```python
from build123d import *

# Parameters (mm, degrees)
F1_DEPTH = 2.413
F2_R     = 10.922
F3_DEPTH = 1.524
F4_R     = 6.223
F4_R_2   = 1.27
F5_DEPTH = 12.065
F6_R     = 5.461
F6_R_2   = 1.524
F7_DEPTH = 1.27


with BuildPart() as f1:
    # F0 (on Top) → F1 (new body)
    with BuildSketch(Plane.XY):
        with BuildLine():
            Line((-16.002, -18.188851), (16.002, -18.188851))
            Line((16.002, -18.188851), (16.002, 18.188851))
            Line((16.002, 18.188851), (9.906, 18.188851))
            Line((9.906, 18.188851), (9.906, 4.600136))
            ThreePointArc((9.906, 4.600136), (5.875687, 9.206866), (0, 10.922))
            ThreePointArc((0, 10.922), (-5.875687, 9.206866), (-9.906, 4.600136))
            Line((-9.906, 4.600136), (-9.906, 18.188851))
            Line((-9.906, 18.188851), (-16.002, 18.188851))
            Line((-16.002, 18.188851), (-16.002, -18.188851))
        make_face()
    extrude(amount=F1_DEPTH)

    # F2 (on face) → F3 (join)
    with BuildSketch(Plane(origin=(0, 0, 0), x_dir=(1, 0, 0), z_dir=(0, 0, -1))):
        Circle(F2_R)
    extrude(amount=F3_DEPTH)

    # F4 (on face) → F5 (join)
    with BuildSketch(Plane(origin=(0, 0, -1.524), x_dir=(1, 0, 0), z_dir=(0, 0, -1))):
        Circle(F4_R)
        Circle(F4_R_2, mode=Mode.SUBTRACT)
    extrude(amount=F5_DEPTH)

    # F6 (on face) → F7 (join)
    with BuildSketch(Plane(origin=(0, 0, -13.589), x_dir=(1, 0, 0), z_dir=(0, 0, -1))):
        Circle(F6_R)
        Circle(F6_R_2, mode=Mode.SUBTRACT)
    extrude(amount=F7_DEPTH)


solid = f1.part
```
Part model, mm, in its own coordinate system. A direction names the side the tool comes from. Round coordinates to 2 decimals unless told otherwise and drop trailing zeros. Loops run counter-clockwise (first coordinate to the right, second up) from the corner with the lowest first, then second, coordinate; pieces in that order, holes last.
Item 1: 3-axis set-ups, long thin cutter, end or side, ignore diameter. For faces 1 (the face through (9.906, 11, 1)), 2 (the face through (-0.17, -1.26, -7.47)): which of +Z, -Z, +X, -X, +Y, -Y reach the whole face in a straight line?
Item 2: Cut at A-A, the plane y = 0. Give the cut face in (x, z), then the cut area to 3 significant figures.
Item 3: Mould opens along X. For faces 3 (the face through (5, 5, -1.524)), 4 (the face through (-0.2, -1.51, -14.22)), 5 (the face through (-1.349, 6.075, -7.472)) say: +X half, -X half, draft (parallel to the pull), parting line (faces both ways), or undercut.
Item 4: Cut at C-C, the plane x = 4.5. Give the cut face in (y, z).
Item 5: Drop flat-ended pins along their axis: P1, Ø0.9, axis at x = 0, y = 0.5, coming from the -Z side; P2, Ø3, axis at x = 7, z = -6.5, coming from the +Y side; P3, Ø3, axis at y = -6, z = -5.5, coming from the -X side. Give the stop position or say it passes through.
Item 6: Cut at B-B, the plane y = 15. Give the cut face in (x, z).
Item 7: Cut at D-D, the plane y = 8.5. Give the cut face in (x, z).
Item 8: Drill centre lines: line 1 (X direction, y = 0, z = -9); line 2 (X direction, y = 0, z = -13.85). Where is each one in solid material? Low to high.
A:
1. face 1: +Z, -Z, +Y
1. face 2: -Z
2. outline: (-16, 0) - (-10.92, 0) - (-10.92, -1.52) - (-6.22, -1.52) - (-6.22, -13.59) - (-5.46, -13.59) - (-5.46, -14.86) - (-1.52, -14.86) - (-1.52, -13.59) - (-1.27, -13.59) - (-1.27, -1.52) - (1.27, -1.52) - (1.27, -13.59) - (1.52, -13.59) - (1.52, -14.86) - (5.46, -14.86) - (5.46, -13.59) - (6.22, -13.59) - (6.22, -1.52) - (10.92, -1.52) - (10.92, 0) - (16, 0) - (16, 2.41) - (-16, 2.41) - close
2. area: 240 mm2
3. face 3: draft
3. face 4: undercut
3. face 5: parting line
4. outline: (-18.19, 0) - (-9.95, 0) - (-9.95, -1.52) - (-4.3, -1.52) - (-4.3, -13.59) - (-3.09, -13.59) - (-3.09, -14.86) - (3.09, -14.86) - (3.09, -13.59) - (4.3, -13.59) - (4.3, -1.52) - (9.95, -1.52) - (9.95, 2.41) - (-18.19, 2.41) - close
5. P1: stops at z = -1.52
5. P2: stops at y = 2.91
5. P3: stops at x = -4.3
6. outline: (-16, 0) - (-9.91, 0) - (-9.91, 2.41) - (-16, 2.41) - close; (9.91, 0) - (16, 0) - (16, 2.41) - (9.91, 2.41) - close
7. outline: (-16, 0) - (-9.91, 0) - (-9.91, 2.41) - (-16, 2.41) - close; (-6.86, -1.52) - (6.86, -1.52) - (6.86, 2.41) - (-6.86, 2.41) - close; (9.91, 0) - (16, 0) - (16, 2.41) - (9.91, 2.41) - close
8. line 1: x = -6.22 to -1.27, 1.27 to 6.22
8. line 2: x = -5.46 to -1.52, 1.52 to 5.46
